Could you check a few things on this drawing? It's one solid part, dimensions in mm from its lowest x, y, z. Give positions to 0.01 mm unless a question says otherwise; leave off trailing zeros. Order: outer loops, then holes, each group sorted by start corner. A loop starts at its lowest first (then second) coordinate and runs counter-clockwise, first axis right, second up.
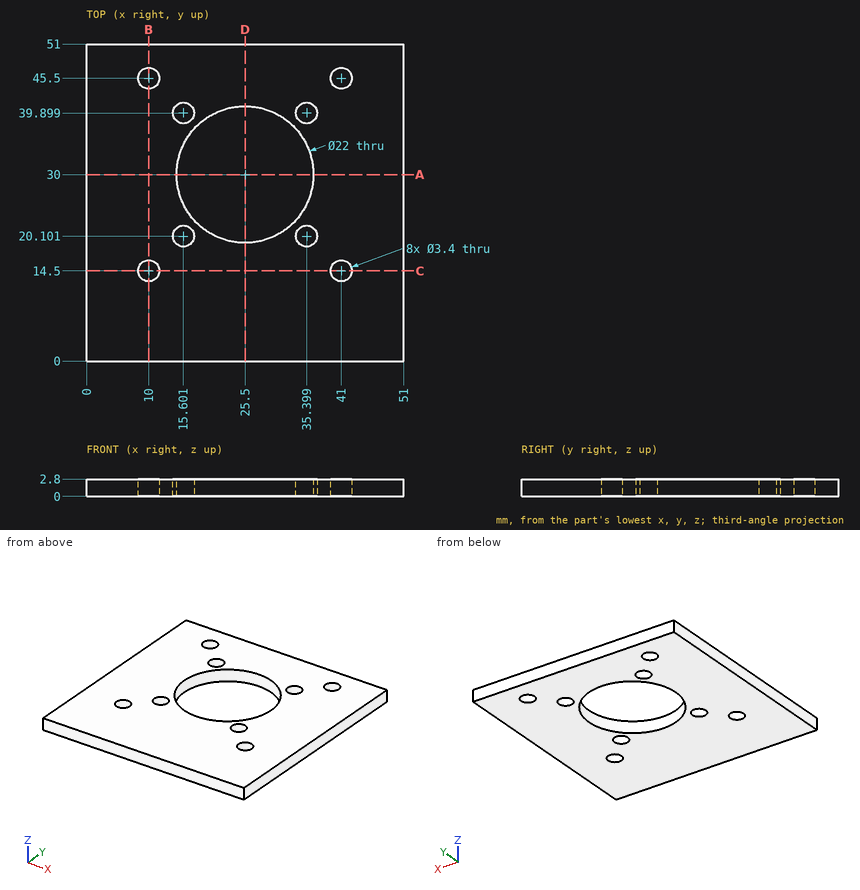
Q1. I need wall thicknesses on L1, parallel to Y at x = 41, z = 2.05; L2, parallel to Y at x = 9.5, z = 1 (1 decimal); L3, parallel to Y at x = 26, z = 0.85. Which ranges of each line are inside material? Lowest first, please.
Filled sheet:
L1: y = 0 to 12.8, 16.2 to 43.8, 47.2 to 51
L2: y = 0 to 12.9, 16.1 to 43.9, 47.1 to 51
L3: y = 0 to 19.01, 40.99 to 51
Q2. If we section it at D-D on x = 25.5: List the corners of the cut face in (y, z) for me.
Filled sheet:
outline: (0, 0) - (19, 0) - (19, 2.8) - (0, 2.8) - close; (41, 0) - (51, 0) - (51, 2.8) - (41, 2.8) - close
Q3. If we section it at A-A on y = 30: List the corners of the cut face in (x, z) for me.
Filled sheet:
outline: (0, 0) - (14.5, 0) - (14.5, 2.8) - (0, 2.8) - close; (36.5, 0) - (51, 0) - (51, 2.8) - (36.5, 2.8) - close
Q4. I'm going to push a flat-ended pin straight in: P1, Ø3, axis at x = 41, y = 14.5, coming from the +Z side. Where does the tip first touch, or does it pass through?
Filled sheet:
P1: passes through
Q5. If we section it at C-C on y = 14.5: List the corners of the cut face in (x, z) for me.
Filled sheet:
outline: (0, 0) - (8.3, 0) - (8.3, 2.8) - (0, 2.8) - close; (11.7, 0) - (39.3, 0) - (39.3, 2.8) - (11.7, 2.8) - close; (42.7, 0) - (51, 0) - (51, 2.8) - (42.7, 2.8) - close
Q6. If we section it at B-B on x = 10: List the corners of the cut face in (y, z) for me.
Filled sheet:
outline: (0, 0) - (12.8, 0) - (12.8, 2.8) - (0, 2.8) - close; (16.2, 0) - (43.8, 0) - (43.8, 2.8) - (16.2, 2.8) - close; (47.2, 0) - (51, 0) - (51, 2.8) - (47.2, 2.8) - close
